Work out the finished part from the listing and answer in its coordinate system (mm). Round coordinates to 2 decimals unless told otherwise and drop trailing zeros. Write each loop counter-clockwise with the first axis right and the second up, starting at its lowest first coordinate (ties: lowest second). Pieces come first, ordered by that corner, then holes. Notation, with made-up numbers: (20.5, 60.25) -> (26.5, 60.25) arc R21 cw to (26.5, 79.25) -> close; hole circle Ø9 at (47, -11). An arc over 180 degrees is marked (long way). One line per item, written item: value.
Autodesk Inventor part; units mm, degrees
ref_plane "YZ Plane" through (0, 0, 0) normal (1, 0, 0) x (0, 1, 0)
ref_plane "XZ Plane" through (0, 0, 0) normal (0, 1, 0) x (-1, 0, 0)
ref_plane "XY Plane" through (0, 0, 0) normal (0, 0, 1) x (1, 0, 0)
sketch "Sketch1" plane through (0, 0, 0) normal (1, 0, 0) x (0, 1, 0)
  circle A0 centre (0, 0) radius 6.35
  dimension "d0" = 12.7
extrude "Extrusion1" add sketch "Sketch1" along normal blind 304.8
sketch "Sketch2" plane through (304.8, 0, 0) normal (1, 0, 0) x (0, 0, -1)
  circle A0 centre (0, 0) radius 4.7625
  circle A1 centre (0, 0) radius 6.35
  dimension "d3" = 9.525
extrude "Extrusion2" cut sketch "Sketch2" against normal blind 385.2875
sketch "Sketch3" plane through (304.8, 0, 0) normal (1, 0, 0) x (0, 0, -1)
  circle A0 centre (0, 0) radius 3.175
  circle A1 centre (0, 0) radius 4.7625
  dimension "d6" = 6.35
extrude "Extrusion3" cut sketch "Sketch3" against normal blind 818.675
properties part number "Guide Shaft" material "Steel, Carbon"
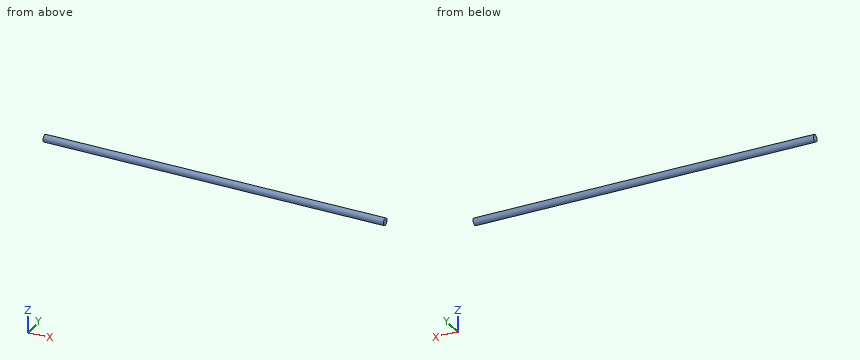
(1) Find section B-B on y = 2. Give the vertices of the cut face in (x, z).
Reported:
outline: (0, -2.47) -> (304.8, -2.47) -> (304.8, 2.47) -> (0, 2.47) -> close
(2) Find section A-A on x = 285.5. Give the vertices of the cut face in (y, z) (3 decimals).
Reported:
outline: circle Ø6.35 at (0, 0)
(3) Consider probe 1 along Z at (x, y) = (127, -0.25); probe 2 along Y at (x, z) = (34.5, 0.5); probe 3 along Z at (x, y) = (210, 1). Determine where each line is inside the solid, lowest interval first.
Reported:
probe 1: z = -3.17 to 3.17
probe 2: y = -3.14 to 3.14
probe 3: z = -3.01 to 3.01
